The model under review builds one solid part; all positions refer to its coordinate system, in mm. Round coordinates to 2 decimals unless told otherwise and drop trailing zeros. Write each loop counter-clockwise with the first axis right and the second up, starting at its lowest first coordinate (ties: lowest second). Pieces come first, ordered by that corner, then holes. Notation, with made-up numbers: (-12.75, 57.5) -> (-0.75, 57.5) arc R30 ccw to (-0.75, 93.5) -> close; hole circle Ø10 at (46, 24.5). An arc over 180 degrees is marked (long way). Use CSV: the item, a comma, the result in double quotes. Start each with the question number.
1) Take a section at A-A, the plane y = 3. Give the boundary of the cut face in (x, z).
2) Take a section at B-B, the plane x = 2.5. Give the boundary of the cut face in (y, z).
3) Wall thickness on probe 1 along Y at (x, z) = (2.5, 0.75); probe 2 along X at (y, z) = (6, 1.25); probe 3 along Y at (x, z) = (2, 0.9): over which ranges is each line inside the solid? List them lowest first. Write a range as [from, to].
4) Take a section at C-C, the plane z = 1.2. Give the boundary of the cut face in (x, y).
5) Mouldability with a two-part tool opening along X and no side actions: class faces 1 (the face through (0, 17, 1)), 2 (the face through (5, 16, 1)), 3 (the face through (9.9, 32.6, 0.3)), 4 (the face through (3.237, 3.676, 0.74)) as released by +X, released by -X, zero draft, split by the parting line, or undercut.
6) For pin 1 Ø0.8 at (y, z) = (34, 1) entering from +X, flat-tipped, find the tip position at first contact; note if it passes through.
7) Take a section at D-D, the plane x = 10.5. Give the boundary of the cut face in (y, z).
from build123d import *

# Parameters (mm, degrees)
SKETCH1_W               = 5
SKETCH1_H               = 1.5
BOSS_EXTRUDE1_DEPTH     = 35
SKETCH2_R               = 1
CUT_EXTRUDE1_DEPTH      = 1
CUT_EXTRUDE1_DEPTH_BACK = 2.5
SKETCH3_R               = 0.75
BOSS_EXTRUDE2_DEPTH     = 10


with BuildPart() as part:
    # Sketch1 → Boss-Extrude1 (new body)
    with BuildSketch(Plane(origin=(0, 0, 0), x_dir=(1, 0, 0), z_dir=(0, 1, 0))):
        with Locations((2.5, -0.75)):
            Rectangle(SKETCH1_W, SKETCH1_H)
    extrude(amount=BOSS_EXTRUDE1_DEPTH)

    # Sketch2 → Cut-Extrude1 (cut, two sides)
    with BuildSketch(Plane(origin=(0, 0, 0), x_dir=(-1, 0, 0), z_dir=(0, 0, -1))) as cut_extrude1_sk:
        with Locations((-2.5, 3)):
            Circle(SKETCH2_R)
    extrude(amount=CUT_EXTRUDE1_DEPTH, mode=Mode.SUBTRACT)
    extrude(cut_extrude1_sk.sketch, amount=-CUT_EXTRUDE1_DEPTH_BACK, mode=Mode.SUBTRACT)

    # Sketch3 → Boss-Extrude2 (add)
    with BuildSketch(Plane(origin=(5, 0, 0), x_dir=(0, 0, -1), z_dir=(1, 0, 0))):
        with Locations((-0.75, 32)):
            Circle(SKETCH3_R)
    extrude(amount=BOSS_EXTRUDE2_DEPTH)


solid = part.part
Values found:
1,outline,"(0, 0) -> (1.5, 0) -> (1.5, 1.5) -> (0, 1.5) -> close; (3.5, 0) -> (5, 0) -> (5, 1.5) -> (3.5, 1.5) -> close"
2,outline,"(0, 0) -> (2, 0) -> (2, 1.5) -> (0, 1.5) -> close; (4, 0) -> (35, 0) -> (35, 1.5) -> (4, 1.5) -> close"
3,probe 1,"[0, 2], [4, 35]"
3,probe 2,"[0, 5]"
3,probe 3,"[0, 2.13], [3.87, 35]"
4,outline,"(0, 0) -> (5, 0) -> (5, 31.4) -> (15, 31.4) -> (15, 32.6) -> (5, 32.6) -> (5, 35) -> (0, 35) -> close; hole circle Ø2 at (2.5, 3)"
5,face 1,"released by -X"
5,face 2,"released by +X"
5,face 3,"zero draft"
5,face 4,"undercut"
6,pin 1,"x = 5"
7,outline,"circle Ø1.5 at (32, 0.75)"
